from build123d import *

# Parameters (mm, degrees)
RESSALTO_EXTRUS_O1_DEPTH = 2


with BuildPart() as part:
    # Esboço1 → Ressalto-extrusão1 (new body)
    with BuildSketch(Plane(origin=(0, 0, 0), x_dir=(0, 0, -1), z_dir=(1, 0, 0))):
        with BuildLine():
            Line((1, 0), (13.619955174, 0))
            ThreePointArc((13.619955174, 0), (14.20826651, -0.191365489), (14.571412872, -0.692220455))
            Line((14.571412872, -0.692220455), (15.270830572, -2.854373095))
            Line((15.270830572, -2.854373095), (18.125203668, -1.931034461))
            ThreePointArc((18.125203668, -1.931034461), (18.8881324, -1.992076966), (19.384440911, -2.574712615))
            Line((19.384440911, -2.574712615), (19.692220455, -3.526170314))
            ThreePointArc((19.692220455, -3.526170314), (19.631177951, -4.289099046), (19.048542302, -4.785407557))
            Line((19.048542302, -4.785407557), (16.194169206, -5.708746191))
            Line((16.194169206, -5.708746191), (17.269391177, -9.032645519))
            ThreePointArc((17.269391177, -9.032645519), (17.200620929, -9.810385556), (16.593756544, -10.301633488))
            ThreePointArc((16.593756544, -10.301633488), (12.880660395, -11.123916543), (9.094724575, -11.484364042))
            ThreePointArc((9.094724575, -11.484364042), (8.366122719, -11.203742859), (8.061318263, -10.484922189))
            Line((8.061318263, -10.484922189), (8.061318263, -5.79672436))
            ThreePointArc((8.061318263, -5.79672436), (7.061318263, -4.79672436), (6.061318263, -5.79672436))
            Line((6.061318263, -5.79672436), (6.061318263, -8.79672436))
            ThreePointArc((6.061318263, -8.79672436), (5.768425044, -9.503831141), (5.061318263, -9.79672436))
            Line((5.061318263, -9.79672436), (1, -9.79672436))
            ThreePointArc((1, -9.79672436), (0.292893219, -9.503831141), (0, -8.79672436))
            Line((0, -8.79672436), (0, -1))
            ThreePointArc((0, -1), (0.292893219, -0.292893219), (1, 0))
        make_face()
    extrude(amount=RESSALTO_EXTRUS_O1_DEPTH)


solid = part.part
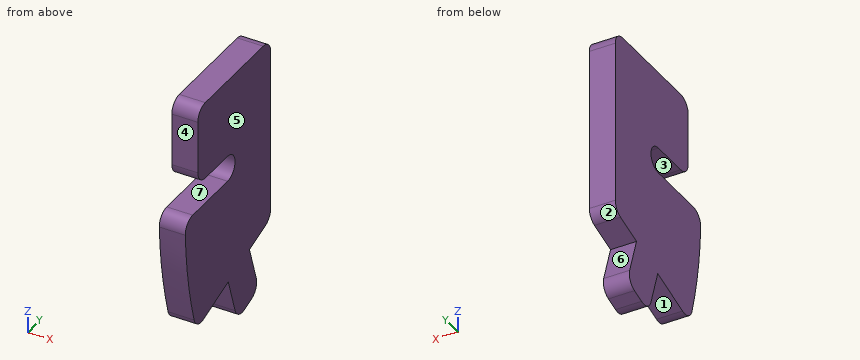
For this review, take the finished solid that the model builds, in its own axes (mm). Face numbers are marked on the shaded views. A direction names the side the tool comes from. Coordinates: 2 decimals unless noted, no trailing zeros. Loops run counter-clockwise (first coordinate to the right, second up) from the corner with the lowest first, then second, coordinate; pieces in that order, holes last. Notation, with made-up numbers: (8, 61) - (57, 61) arc R16 cw to (57, 73) - close; hole circle Ø10 at (28, -34). An arc over 180 degrees is marked (long way). Return JSON: item names as keys, results as strings.
Item 1: Take a section at A-A (y = -7.75). Give the boundary of the cut face in (x, z).
Determined:
{"outline": "(0, -16.85) - (2, -16.85) - (2, -8.06) - (0, -8.06) - close; (0, -6.06) - (2, -6.06) - (2, 0) - (0, 0) - close"}
Item 2: For the marked faces 4, 5, 6 and 7, list the 3-axis set-ups (+Z, -Z, +X, -X, +Y, -Y) from which the entire face can be reached by the end or side of a thin tool; tool diameter is ignored.
Determined:
{"face 4": "+Z, +X, -X, -Y", "face 5": "+Z, -Z, +X, +Y, -Y", "face 6": "+X, -X, +Y", "face 7": "+X, -X, -Y"}
Item 3: Mouldability with a two-part tool opening along Y and no side actions: class the marked faces 1, 2 and 3 as pulls with the +Y half, pulls with the -Y half, needs draft (parallel to the pull), parting line crosses it, or undercut.
Determined:
{"face 1": "undercut", "face 2": "pulls with the +Y half", "face 3": "needs draft"}
Item 4: For line 1 (Y direction, x = 1.8, z = -7); line 2 (Y direction, x = 1.05, z = -5); line 3 (Z direction, x = 1.2, y = -9.5), list the stretches that pass through material, from the lowest coordinate up.
Determined:
{"line 1": "y = -4.8 to 0", "line 2": "y = -9.8 to 0", "line 3": "z = -17.31 to -8.06, -5.77 to -0.29"}
Item 5: Insertion check: pin 1 (1 mm diameter, centred on x = 1.5, y = -7.5, fed in from -Z); pin 2 (0.6 mm diameter, centred on x = 1, z = -2.5, fed in from -Y). Each pin has a flat end and moves straight along its axis. Give the tip position at first contact, or say it passes through.
Determined:
{"pin 1": "stops at z = -16.94", "pin 2": "stops at y = -9.8"}
Item 6: Take a section at C-C (y = -6.5). Give the boundary of the cut face in (x, z), then the cut area to 3 significant figures.
Determined:
{"outline": "(0, -16.45) - (2, -16.45) - (2, -8.06) - (0, -8.06) - close; (0, -6.06) - (2, -6.06) - (2, 0) - (0, 0) - close", "area": "28.9 mm2"}
Item 7: Take a section at B-B (x = 1.7). Give the boundary of the cut face in (y, z), then the cut area to 3 significant figures.
Determined:
{"outline": "(-11.48, -9.09) arc R30.93 ccw to (-10.3, -16.59) arc R1 ccw to (-9.03, -17.27) - (-5.71, -16.19) - (-4.79, -19.05) arc R1 ccw to (-3.53, -19.69) - (-2.57, -19.38) arc R1 ccw to (-1.93, -18.13) - (-2.85, -15.27) - (-0.69, -14.57) arc R1 ccw to (0, -13.62) - (0, -1) arc R1 ccw to (-1, 0) - (-8.8, 0) arc R1 ccw to (-9.8, -1) - (-9.8, -5.06) arc R1 ccw to (-8.8, -6.06) - (-5.8, -6.06) arc R1 cw to (-5.8, -8.06) - (-10.48, -8.06) arc R1 ccw to start", "area": "168 mm2"}
Item 8: Take a section at D-D (z = -17.75). Give the boundary of the cut face in (x, y), then the cut area to 3 significant figures.
Determined:
{"outline": "(0, -5.21) - (2, -5.21) - (2, -2.05) - (0, -2.05) - close", "area": "6.31 mm2"}
